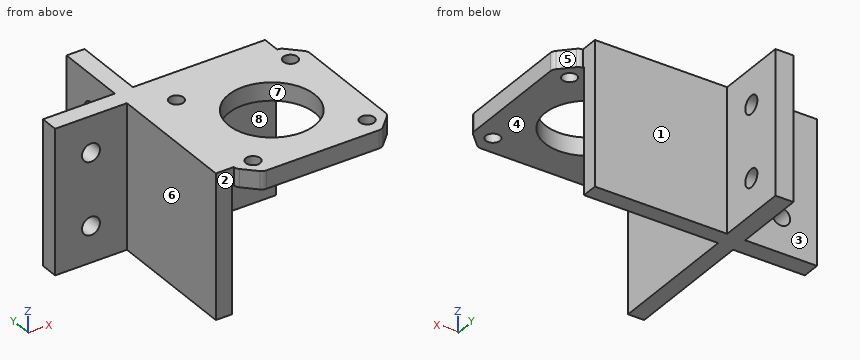
Autodesk Inventor part; units mm, degrees
ref_plane "YZ Plane" through (0, 0, 0) normal (1, 0, 0) x (0, 1, 0)
ref_plane "XZ Plane" through (0, 0, 0) normal (0, 1, 0) x (-1, 0, 0)
ref_plane "XY Plane" through (0, 0, 0) normal (0, 0, 1) x (1, 0, 0)
sketch "Sketch1" plane through (0, 0, 0) normal (0, 0, 1) x (1, 0, 0)
  arc A0 (-20.5392, 17.1146) -> (-21.125, 15.7004) centre (-19.125, 15.7004) ccw
  line L0 (-21.125, -15.7004) -> (-21.125, 15.7004)
  arc A1 (-21.125, -15.7004) -> (-20.5392, -17.1146) centre (-19.125, -15.7004) ccw
  line L1 (-20.5392, -17.1146) -> (-17.1146, -20.5392)
  arc A2 (-17.1146, -20.5392) -> (-15.7004, -21.125) centre (-15.7004, -19.125) ccw
  line L2 (15.7004, -21.125) -> (-15.7004, -21.125)
  arc A3 (15.7004, -21.125) -> (17.1146, -20.5392) centre (15.7004, -19.125) ccw
  line L3 (20.5392, -17.1146) -> (17.1146, -20.5392)
  arc A4 (20.5392, -17.1146) -> (21.125, -15.7004) centre (19.125, -15.7004) ccw
  line L4 (21.125, 15.7004) -> (21.125, -15.7004)
  arc A5 (21.125, 15.7004) -> (20.5392, 17.1146) centre (19.125, 15.7004) ccw
  line L5 (20.5392, 17.1146) -> (17.1146, 20.5392)
  arc A6 (17.1146, 20.5392) -> (15.7004, 21.125) centre (15.7004, 19.125) ccw
  line L6 (-15.7004, 21.125) -> (15.7004, 21.125)
  arc A7 (-15.7004, 21.125) -> (-17.1146, 20.5392) centre (-15.7004, 19.125) ccw
  line L7 (-20.5392, 17.1146) -> (-17.1146, 20.5392)
  circle A8 centre (0, 0) radius 16
  circle A9 centre (-15.875, -15.875) radius 1.625
  circle A10 centre (15.875, 15.875) radius 1.625
  circle A11 centre (-15.875, 15.875) radius 1.625
  circle A12 centre (15.875, -15.875) radius 1.625
  circle A13 centre (0, 0) radius 12
  circle A14 centre (-15.875, 15.875) radius 2
  circle A15 centre (15.875, 15.875) radius 2
  circle A16 centre (15.875, -15.875) radius 2
  circle A17 centre (-15.875, -15.875) radius 2
  point P0 (0, 0)
  dimension "d0" = 24
  dimension "d1" = 4
  dimension "d2" = 4
  dimension "d3" = 4
  dimension "d4" = 4
extrude "Extrusion1" add sketch "Sketch1" along normal blind 5 contours L7 A7 L6 A6 L5 A5 L4 A4 L3 A3 L2 A2 L1 A1 L0 A0 | A8
sketch "Sketch3" plane through (0, 0, 5) normal (0, 0, 1) x (1, 0, 0)
  line L0 (-15.7004, 21.125) -> (15.7004, 21.125)
  line L1 (15.7004, 21.125) -> (-46.125, 21.125)
  line L2 (-46.125, 21.125) -> (-46.125, 26.125)
  line L3 (-46.125, 26.125) -> (15.7004, 26.125)
  line L4 (15.7004, 26.125) -> (15.7004, 21.125)
  line L5 (-21.125, 15.7004) -> (-21.125, -15.7004)
  line L6 (-21.125, -15.7004) -> (-26.125, -15.7004)
  line L7 (-26.125, -15.7004) -> (-26.125, 46.125)
  line L8 (-26.125, 46.125) -> (-21.125, 46.125)
  line L9 (-21.125, 46.125) -> (-21.125, -15.7004)
  point P0 (0, 0)
  dimension "d11" = 5
  dimension "d12" = 5
  dimension "d13" = 20
  dimension "d14" = 20
extrude "Extrusion3" add sketch "Sketch3" against normal blind 40
sketch "Sketch4" plane through (0, 0, 5) normal (0, 0, 1) x (1, 0, 0)
  arc A0 (-15.7004, 21.125) -> (-17.1146, 20.5392) centre (-15.7004, 19.125) ccw
  line L0 (-17.1146, 20.5392) -> (-20.5392, 17.1146)
  arc A1 (-20.5392, 17.1146) -> (-21.125, 15.7004) centre (-19.125, 15.7004) ccw
  line L1 (-21.125, 21.125) -> (-21.125, 15.7004)
  line L2 (-15.7004, 21.125) -> (-21.125, 21.125)
  circle A2 centre (0, 0) radius 12
  circle A3 centre (-15.875, -15.875) radius 2
  circle A4 centre (15.875, -15.875) radius 2
  circle A5 centre (15.875, 15.875) radius 2
  circle A6 centre (-15.875, 15.875) radius 2
  line L3 (15.7004, 26.125) -> (15.7004, 21.125)
  line L4 (-21.125, 26.125) -> (15.7004, 26.125)
  line L5 (-21.125, 46.125) -> (-21.125, 26.125)
  line L6 (-26.125, 46.125) -> (-21.125, 46.125)
  line L7 (-26.125, 26.125) -> (-26.125, 46.125)
  line L8 (-46.125, 26.125) -> (-26.125, 26.125)
  line L9 (-46.125, 21.125) -> (-46.125, 26.125)
  line L10 (-26.125, 21.125) -> (-46.125, 21.125)
  line L11 (-26.125, -15.7004) -> (-26.125, 21.125)
  line L12 (-21.125, -15.7004) -> (-26.125, -15.7004)
  arc A7 (-21.125, -15.7004) -> (-20.5392, -17.1146) centre (-19.125, -15.7004) ccw
  line L13 (-20.5392, -17.1146) -> (-17.1146, -20.5392)
  arc A8 (-17.1146, -20.5392) -> (-15.7004, -21.125) centre (-15.7004, -19.125) ccw
  line L14 (-15.7004, -21.125) -> (15.7004, -21.125)
  arc A9 (15.7004, -21.125) -> (17.1146, -20.5392) centre (15.7004, -19.125) ccw
  line L15 (17.1146, -20.5392) -> (20.5392, -17.1146)
  arc A10 (20.5392, -17.1146) -> (21.125, -15.7004) centre (19.125, -15.7004) ccw
  line L16 (21.125, -15.7004) -> (21.125, 15.7004)
  arc A11 (21.125, 15.7004) -> (20.5392, 17.1146) centre (19.125, 15.7004) ccw
  line L17 (20.5392, 17.1146) -> (17.1146, 20.5392)
  arc A12 (17.1146, 20.5392) -> (15.7004, 21.125) centre (15.7004, 19.125) ccw
  point P0 (0, 0)
extrude "Extrusion4" add sketch "Sketch4" against normal blind 5 contours A0 L0 A1 L1 L2
sketch "Sketch5" plane through (-21.125, 26.125, 5) normal (1, 0, 0) x (0, 0, -1)
  circle A0 centre (10, 10) radius 2.5
  circle A1 centre (30, 10) radius 2.5
  line L0 (0, 20) -> (40, 20)
  line L1 (0, 20) -> (0, 0)
  point P0 (5, -26.125)
  dimension "d19" = 5
  dimension "d20" = 5
  dimension "d21" = 10
  dimension "d22" = 10
  dimension "d23" = 20
  dimension "d24" = 10
extrude "Extrusion5" cut sketch "Sketch5" against normal through all
sketch "Sketch6" plane through (-46.125, 21.125, 5) normal (0, -1, 0) x (1, 0, 0)
  circle A0 centre (10, -30) radius 2.5
  circle A1 centre (10, -10) radius 2.5
  line L0 (0, 0) -> (0, -40)
  line L1 (20, 0) -> (0, 0)
  point P0 (46.125, -5)
  dimension "d27" = 10
  dimension "d28" = 10
  dimension "d29" = 5
  dimension "d30" = 5
  dimension "d31" = 20
  dimension "d32" = 10
extrude "Extrusion6" cut sketch "Sketch6" against normal through all
sketch "Sketch7" plane through (0, 0, -35) normal (0, 0, -1) x (-1, 0, 0)
  line L0 (21.625, 21.625) -> (-23.2924, 21.625)
  line L1 (-23.2924, 21.625) -> (-23.2924, -21.9013)
  line L2 (-23.2924, -21.9013) -> (21.625, -21.9013)
  line L3 (21.625, -21.9013) -> (21.625, 21.625)
  line L4 (-15.7004, 21.125) -> (21.125, 21.125)
  line L5 (21.125, 21.125) -> (21.125, -15.7004)
  point P0 (0, 0)
  dimension "d35" = 0.5
  dimension "d36" = 0.5
extrude "Extrusion7" cut sketch "Sketch7" against normal blind 35
equation "\"d36\" = d35"
properties part number "StepperXYHolder"
Geometry check sheet. Reference: the model listing, model coordinates, mm. Face numbers are marked on the shaded views. A direction names the side the tool comes from. Coordinates: 2 decimals unless noted, no trailing zeros. Order: outer loops, then holes, each group sorted by start corner. A loop starts at its lowest first (then second) coordinate and runs counter-clockwise, first axis right, second up. Notation, with made-up numbers: (73.5, 38) - (110.5, 38) arc R18 ccw to (110.5, 46) - close; hole circle Ø1 at (47, 84.5). An arc over 180 degrees is marked (long way). Answer in a Markdown table with one row per item. Add a question column.
1) Gauge pin test, flat ends, axial feed: P1, Ø4, axis at x = -22.5, z = -13, coming from the -Y side; P2, Ø16, axis at y = 41, z = -22.5, coming from the -X side (3 decimals); P3, Ø6, axis at y = 38, z = -21, coming from the +X side (3 decimals). Record the tip position at first contact, or that the pin passes through.
2) Cross-section at B-B, the plane x = 0. Record the cut outline in (y, z) (3 decimals).
3) Cross-section at A-A, the plane z = -25. Record the cut outline in (x, y) (3 decimals).
4) Release check for a two-part mould opening along X. For the marked faces 5, 6, 7 and 8 record: +X half, -X half, draft (parallel to the pull), parting line (faces both ways), or undercut.
5) Material ranges on line 1 along Y through (x, z) = (-2, -4.5) (3 decimals); line 2 along Y through (x, z) = (-23.5, -33) (3 decimals); line 3 along X through (y, z) = (20, -21) (3 decimals), recorded low to high. Write a range as [from, to].
6) Cross-section at D-D, the plane z = -12.5. Record the cut outline in (x, y) (3 decimals).
7) Set-up check for the marked faces 1, 2, 3 and 4: record each of +Z, -Z, +X, -X, +Y, -Y from which the full face is reachable in a straight line by a thin tool's end or side.
8) Cross-section at C-C, the plane y = 0. Record the cut outline in (x, z) (3 decimals).
Check result:
| question | item | result |
|---|---|---|
| 1 | P1 | stops at y = -15.7 |
| 1 | P2 | stops at x = -26.125 |
| 1 | P3 | stops at x = -21.125 |
| 2 | outline | (-21.125, 0) - (-12, 0) - (-12, 5) - (-21.125, 5) - close; (12, 0) - (21.625, 0) - (21.625, -35) - (26.125, -35) - (26.125, 5) - (12, 5) - close |
| 3 | outline | (-46.125, 21.125) - (-38.625, 21.125) - (-38.625, 26.125) - (-46.125, 26.125) - close; (-33.625, 21.125) - (-26.125, 21.125) - (-26.125, -15.7) - (-21.625, -15.7) - (-21.625, 21.625) - (15.7, 21.625) - (15.7, 26.125) - (-21.125, 26.125) - (-21.125, 33.625) - (-26.125, 33.625) - (-26.125, 26.125) - (-33.625, 26.125) - close; (-26.125, 38.625) - (-21.125, 38.625) - (-21.125, 46.125) - (-26.125, 46.125) - close |
| 4 | face 5 | +X half |
| 4 | face 6 | -X half |
| 4 | face 7 | undercut |
| 4 | face 8 | draft |
| 5 | line 1 | y = [21.625, 26.125] |
| 5 | line 2 | y = [-15.7, 46.125] |
| 5 | line 3 | x = [-26.125, -21.625] |
| 6 | outline | (-46.125, 21.125) - (-26.125, 21.125) - (-26.125, -15.7) - (-21.625, -15.7) - (-21.625, 21.625) - (15.7, 21.625) - (15.7, 26.125) - (-21.125, 26.125) - (-21.125, 46.125) - (-26.125, 46.125) - (-26.125, 26.125) - (-46.125, 26.125) - close |
| 7 | face 1 | +Z, -Z, +X, +Y |
| 7 | face 2 | +Z, -Z, -X, -Y |
| 7 | face 3 | +Z, -Z, -X, +Y |
| 7 | face 4 | -Z, +X, -Y |
| 8 | outline | (-26.125, -35) - (-21.625, -35) - (-21.625, 0) - (-12, 0) - (-12, 5) - (-26.125, 5) - close; (12, 0) - (21.125, 0) - (21.125, 5) - (12, 5) - close |
